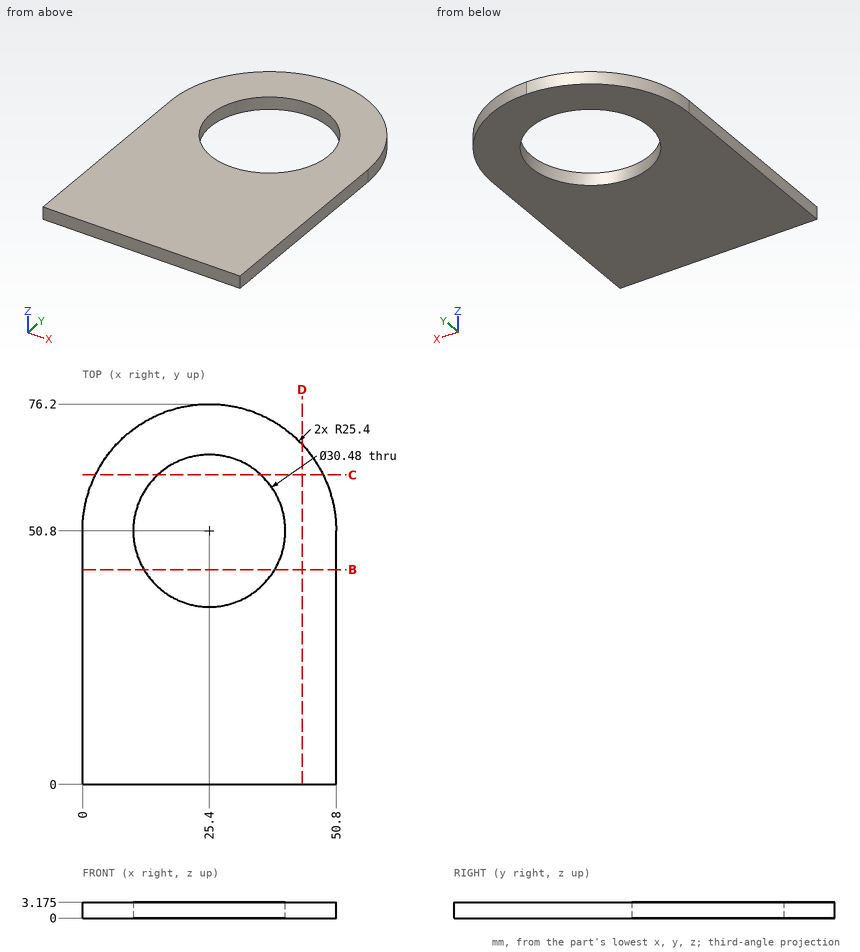
Answer from the drawing. Dimensions are ordinates in mm from the lowest x, y and z of the part. Coordinates: 2 decimals unless noted, no trailing zeros. Loops run counter-clockwise (first coordinate to the right, second up) from the corner with the lowest first, then second, coordinate; pieces in that order, holes last.
Q1. Consider probe 1 along X at (y, z) = (40, 1.9); probe 2 along X at (y, z) = (54.5, 3); probe 3 along Y at (x, z) = (35, 1.9). Determine where each line is inside the solid, lowest interval first.
Q2. The part is cut by section B-B on y = 43. Write down the section's boundary in (x, z) (1 decimal).
Q3. The part is cut by section C-C on y = 62. Write down the section's boundary in (x, z) (1 decimal).
Q4. The part is cut by section D-D on x = 44. Write down the section's boundary in (y, z) (1 decimal).
Results below:
1. probe 1: x = 0 to 14.65, 36.15 to 50.8
1. probe 2: x = 0.27 to 10.62, 40.18 to 50.53
1. probe 3: y = 0 to 38.96, 62.64 to 74.32
2. outline: (0, 0) - (12.3, 0) - (12.3, 3.2) - (0, 3.2) - close; (38.5, 0) - (50.8, 0) - (50.8, 3.2) - (38.5, 3.2) - close
3. outline: (2.6, 0) - (15.1, 0) - (15.1, 3.2) - (2.6, 3.2) - close; (35.7, 0) - (48.2, 0) - (48.2, 3.2) - (35.7, 3.2) - close
4. outline: (0, 0) - (68.1, 0) - (68.1, 3.2) - (0, 3.2) - close
